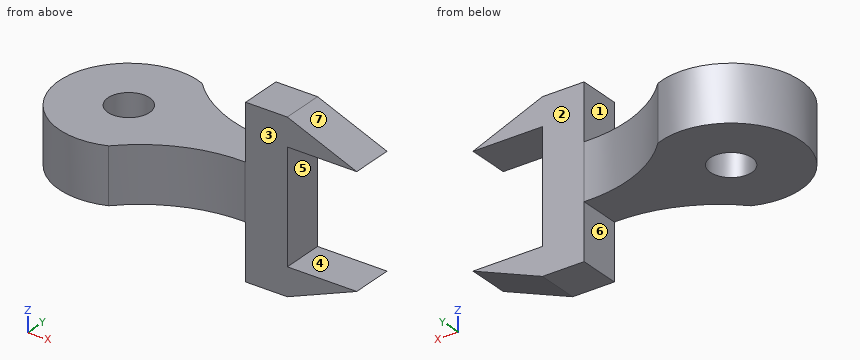
```python
from build123d import *

# Parameters (mm, degrees)
SKETCH1_R           = 15
BOSS_EXTRUDE1_DEPTH = 20
SKETCH5_W           = 30
SKETCH5_H           = 30
BOSS_EXTRUDE2_DEPTH = 60
BOSS_EXTRUDE3_DEPTH = 30


with BuildPart() as part:
    # Sketch1 → Boss-Extrude1 (new, symmetric)
    with BuildSketch(Plane.XY):
        with BuildLine():
            Line((95, 15), (125, 15))
            Line((125, 15), (125, -15))
            Line((125, -15), (94.520902358, -15))
            ThreePointArc((94.520902358, -15), (53.491668614, -22.559030862), (19.11731281, -46.200956169))
            ThreePointArc((19.11731281, -46.200956169), (-50, 0), (19.11731281, 46.200956169))
            ThreePointArc((19.11731281, 46.200956169), (53.711420625, 22.459790206), (95, 15))
        make_face()
        Circle(SKETCH1_R, mode=Mode.SUBTRACT)
    extrude(amount=BOSS_EXTRUDE1_DEPTH, both=True)

    # Sketch5 → Boss-Extrude2 (add, symmetric)
    with BuildSketch(Plane.XY):
        with Locations((110, 0)):
            Rectangle(SKETCH5_W, SKETCH5_H)
    extrude(amount=BOSS_EXTRUDE2_DEPTH, both=True)

    # Sketch6 → Boss-Extrude3 (add)
    with BuildSketch(Plane(origin=(0, 15, 0), x_dir=(1, 0, 0), z_dir=(0, 1, 0))):
        Polygon((125, 60), (175, 40), (125, 40), align=None)
        Polygon((125, -60), (175, -40), (125, -40), align=None)
    extrude(amount=-BOSS_EXTRUDE3_DEPTH)


solid = part.part
```
Verification items for the finished model (mm, model axes). Face numbers are marked on the shaded views. A direction names the side the tool comes from. Coordinates: 2 decimals unless noted, no trailing zeros. Loops run counter-clockwise (first coordinate to the right, second up) from the corner with the lowest first, then second, coordinate; pieces in that order, holes last. Notation, with made-up numbers: (18, -3.75) - (47, -3.75) arc R25 cw to (47, 35.25) - close; hole circle Ø3 at (40.25, -26). An arc over 180 degrees is marked (long way). Answer as a JSON object with one key per item and string values.
(1) Mould release check, pull along Z, two halves, no side actions. Record for the marked faces 5, 6 and 7: pulls with the +Z half, pulls with the -Z half, needs draft (parallel to the pull), parting line crosses it, or undercut.
Response:
{"face 5": "undercut", "face 6": "needs draft", "face 7": "pulls with the +Z half"}
(2) Cross-section at D-D, the plane x = 131. Record the boundary of the cut face in (y, z).
Response:
{"outline": "(-15, -57.6) - (15, -57.6) - (15, -40) - (-15, -40) - close; (-15, 40) - (15, 40) - (15, 57.6) - (-15, 57.6) - close"}
(3) Scan lines: line 1 along Y through (x, z) = (0, 11); line 2 along Z through (x, y) = (-27.5, 17); line 3 along Y through (x, z) = (125, -49). Record each from-to range of solid material in increasing order.
Response:
{"line 1": "y = -50 to -15, 15 to 50", "line 2": "z = -20 to 20", "line 3": "y = -15 to 15"}
(4) Go/stop test with flat-tipped pins: pin 1 Ø6 at (y, z) = (7.5, 38) entering from -X; pin 2 Ø9 at (y, z) = (-7, -12.5) entering from +X; pin 3 Ø15 at (x, y) = (149.5, -3) entering from -Z; pin 4 Ø2 at (x, z) = (43.5, -22.5) entering from -Y. Record where each tip stops, or that it passes through.
Response:
{"pin 1": "stops at x = 95", "pin 2": "stops at x = 125", "pin 3": "stops at z = -53.2", "pin 4": "passes through"}
(5) Access from +Z, -Z, +X, -X, +Y, -Y to the whole of each face (thin tool, end or side, straight path). Record for the marked faces 1, 2, 3 and 4.
Response:
{"face 1": "+Z, -X, +Y, -Y", "face 2": "+Z, -Z, +X, +Y", "face 3": "+Z, -Z, +X, -Y", "face 4": "+X, +Y, -Y"}
(6) Cross-section at C-C, the plane z = -2. Record the boundary of the cut face in (x, y), then the cut area to 3 significant figures.
Response:
{"outline": "(19.12, -46.2) arc R100 cw to (94.52, -15) - (125, -15) - (125, 15) - (95, 15) arc R100 cw to (19.12, 46.2) arc R50 ccw (long way) to start; hole circle Ø30 at (0, 0)", "area": "9,660 mm²"}
(7) Cross-section at B-B, the plane y = 0. Record the boundary of the cut face in (x, z), then the cut area to 3 significant figures.
Response:
{"outline": "(-50, -20) - (-15, -20) - (-15, 20) - (-50, 20) - close; (15, -20) - (95, -20) - (95, -60) - (125, -60) - (175, -40) - (125, -40) - (125, 40) - (175, 40) - (125, 60) - (95, 60) - (95, 20) - (15, 20) - close", "area": "9,200 mm²"}
(8) Cross-section at A-A, the plane x = 0. Record the boundary of the cut face in (y, z), then the cut area to 3 significant figures.
Response:
{"outline": "(-50, -20) - (-15, -20) - (-15, 20) - (-50, 20) - close; (15, -20) - (50, -20) - (50, 20) - (15, 20) - close", "area": "2,800 mm²"}
